from build123d import *

# Parameters (mm, degrees)
BOSS_EXTRUDE1_DEPTH = 177.8
SKETCH2_R           = 2.032
CUT_EXTRUDE1_DEPTH  = 186.827403736
FILLET2_R           = 12.7


with BuildPart() as part:
    # Sketch1 → Boss-Extrude1 (new body)
    with BuildSketch(Plane(origin=(0, 0, 0), x_dir=(1, 0, 0), z_dir=(0, 1, 0))):
        with BuildLine():
            Line((-20.574, -9.652129604), (-4.162019583, -14.39674322))
            ThreePointArc((-4.162019583, -14.39674322), (12.103082443, -8.837647749), (12.446, 8.347796497))
            Line((12.446, 8.347796497), (12.446, 20.746712887))
            Line((12.446, 20.746712887), (31.496, 20.746712887))
            Line((31.496, 20.746712887), (31.496, 17.571712887))
            Line((31.496, 17.571712887), (18.796, 17.571712887))
            Line((18.796, 17.571712887), (18.796, -12.827129604))
            ThreePointArc((18.796, -12.827129604), (-4.064, -19.155968814), (-26.924, -12.827129604))
            Line((-26.924, -12.827129604), (-26.924, 17.571712887))
            Line((-26.924, 17.571712887), (-39.624, 17.571712887))
            Line((-39.624, 17.571712887), (-39.624, 20.746712887))
            Line((-39.624, 20.746712887), (-20.574, 20.746712887))
            Line((-20.574, 20.746712887), (-20.574, 9.652))
            Line((-20.574, 9.652), (-20.574, -9.652129604))
        make_face()
    extrude(amount=BOSS_EXTRUDE1_DEPTH)

    # Sketch2 → Cut-Extrude1 (cut, through all)
    with BuildSketch(Plane.XY.offset(-17.571712887)):
        with Locations((-33.274, 171.45)):
            Circle(SKETCH2_R)
        with Locations((-33.274, 6.35)):
            Circle(SKETCH2_R)
        with Locations((25.146, 171.45)):
            Circle(SKETCH2_R)
        with Locations((25.146, 6.35)):
            Circle(SKETCH2_R)
    extrude(amount=-CUT_EXTRUDE1_DEPTH, mode=Mode.SUBTRACT)

    # Fillet2
    fillet2_edges = [part.edges().sort_by_distance(p)[0] for p in [
        (18.796, 88.9, 12.827129604),
        (-26.924, 88.9, 12.827129604),
    ]]
    fillet(fillet2_edges, radius=FILLET2_R)


solid = part.part
Could you check a few things on this model? Use its own coordinates, in mm. A direction names the side the tool comes from. Round coordinates to 2 decimals unless told otherwise and drop trailing zeros. Write each loop counter-clockwise with the first axis right and the second up, starting at its lowest first coordinate (ties: lowest second). Pieces come first, ordered by that corner, then holes. Notation, with made-up numbers: (-14.5, 57.25) - (6.5, 57.25) arc R21 ccw to (6.5, 71.25) - close; hole circle Ø9 at (35.5, -2.75). An arc over 180 degrees is marked (long way). Put each result on its own line as item: value. Start each with the question number.
(1) Thinking about a two-plate mould opening in Y: for faces 6 (the cylindrical face through (11.95, 87.655, 9.043)), 7 (the cylindrical face through (24.881, 173.465, -19.137)), 8 (the flat face through (-7, 0, 14)), which applies, released by +Y, released by -Y, zero draft, split by the parting line, or undercut?
(2) I want a section at B-B, the plane y = 6.35. Please give me the cut outline in (x, z), plus the area to 3 significant figures.
(3) For faces 1 (the flat face through (-39.624, 88, -19)), 2 (the flat face through (-12.48, 87.66, 11.99)), 3 (the flat face through (-26.924, 88, -6)), 4 (the cylindrical face through (-35.304, 6.439, -19.137)), 5 (the flat face through (18.796, 88, -7)), which set-ups out of +Z, -Z, +X, -X, +Y, -Y let a thin tool reach every point of the face, with its end or its side?
(4) I need wall thicknesses on probe 1 along X at (y, z) = (171.45, -18.9); probe 2 along X at (y, z) = (171, -18); probe 3 along X at (y, z) = (130, -16.5). Which ranges of each line are inside material? Lowest first, please.
(5) Will these pins go through, and if not, where does the flat tip stop? pin 1 (4 mm diameter, centred on x = 24, y = 92.5, fed in from +Z); pin 2 (2 mm diameter, centred on y = 89, z = 13, fed in from -X); pin 3 (1.5 mm diameter, centred on y = 98, z = 0.5, fed in from -X).
(6) I want a section at A-A, the plane z = 12. Please give me the cut outline in (x, y), plus the area to 3 significant figures.
(7) I want a section at D-D, the plane x = -29.5. Please give me the cut outline in (y, z).
(8) I want a section at C-C, the plane y = 164. Please give me the cut outline in (x, z).
Here are the results:
1. face 6: zero draft
1. face 7: undercut
1. face 8: released by -Y
2. outline: (-39.62, -20.75) - (-35.31, -20.75) - (-35.31, -17.57) - (-39.62, -17.57) - close; (-31.24, -20.75) - (-20.57, -20.75) - (-20.57, 9.65) - (-4.16, 14.4) arc R14.99 cw to (12.45, -8.35) - (12.45, -20.75) - (23.11, -20.75) - (23.11, -17.57) - (18.8, -17.57) - (18.8, 4.79) arc R12.7 ccw to (10.16, 16.82) arc R44.45 ccw to (-18.29, 16.82) arc R12.7 ccw to (-26.92, 4.79) - (-26.92, -17.57) - (-31.24, -17.57) - close; (27.18, -20.75) - (31.5, -20.75) - (31.5, -17.57) - (27.18, -17.57) - close
2. area: 626 mm^2
3. face 1: +Z, -Z, -X, +Y, -Y
3. face 2: -Z, +Y, -Y
3. face 3: +Z, -X, +Y, -Y
3. face 4: +Z, -Z
3. face 5: +Z, +X, +Y, -Y
4. probe 1: x = -39.62 to -35.31, -31.24 to -20.57, 12.45 to 23.11, 27.18 to 31.5
4. probe 2: x = -39.62 to -35.26, -31.29 to -20.57, 12.45 to 23.16, 27.13 to 31.5
4. probe 3: x = -26.92 to -20.57, 12.45 to 18.8
5. pin 1: stops at z = -17.57
5. pin 2: stops at x = -24.68
5. pin 3: stops at x = -26.92
6. outline: (-24.68, 0) - (-12.45, 0) - (-12.45, 177.8) - (-24.68, 177.8) - close; (8.98, 0) - (16.55, 0) - (16.55, 177.8) - (8.98, 177.8) - close
6. area: 3,520 mm^2
7. outline: (0, -20.75) - (177.8, -20.75) - (177.8, -17.57) - (0, -17.57) - close
8. outline: (-39.62, -20.75) - (-20.57, -20.75) - (-20.57, 9.65) - (-4.16, 14.4) arc R14.99 cw to (12.45, -8.35) - (12.45, -20.75) - (31.5, -20.75) - (31.5, -17.57) - (18.8, -17.57) - (18.8, 4.79) arc R12.7 ccw to (10.16, 16.82) arc R44.45 ccw to (-18.29, 16.82) arc R12.7 ccw to (-26.92, 4.79) - (-26.92, -17.57) - (-39.62, -17.57) - close
